Read the model definition and answer for the solid it produces. Units are mm, in the model's axes. A direction names the side the tool comes from. Give positions to 0.01 mm unless a question says otherwise; leave off trailing zeros. Write each loop counter-clockwise with the first axis right and the second up, starting at its lowest first coordinate (ties: lowest second). Pieces come first, ordered by that corner, then holes. Notation, with made-up numbers: (52, -3.75) - (74, -3.75) arc R14 cw to (74, 3.25) - close; hole circle Ø4 at (13, 77). An arc over 180 degrees is marked (long way). Answer as CSV lines item,"result".
```python
from build123d import *

# Parameters (mm, degrees)
F0_W      = 115
F0_H      = 60
F1_DEPTH  = 12
F0_W_2    = 12
F2_DEPTH  = 60
F4_DEPTH  = 25
F5_W      = 50
F5_H      = 20
F6_DEPTH  = 48
F8_DEPTH  = 25
F9_R      = 12.5
F10_DEPTH = 25


with BuildPart() as f1:
    # F0 (on Top) → F1 (new body)
    with BuildSketch(Plane.XY):
        with Locations((-0.438802, -3.920759)):
            Rectangle(F0_W, F0_H)
    extrude(amount=F1_DEPTH)

    # F0 (on Top) → F2 (join)
    with BuildSketch(Plane.XY):
        with Locations((63.061198, -3.920759)):
            Rectangle(F0_W_2, F0_H)
    extrude(amount=F2_DEPTH)

    # F3 (on face) → F4 (cut)
    with BuildSketch(Plane.XY.offset(12)):
        Polygon((57.061198, -33.920759), (-57.938802, 6.079241), (-57.938802, -33.920759), align=None)
    extrude(amount=-F4_DEPTH, mode=Mode.SUBTRACT)

    # F5 (on face) → F6 (join)
    with BuildSketch(Plane.XY.offset(12)):
        with Locations((-32.938802, 16.079241)):
            Rectangle(F5_W, F5_H)
    extrude(amount=F6_DEPTH)

    # F7 (on face) → F8 (cut)
    with BuildSketch(Plane.XZ.offset(-6.079241)):
        with BuildLine():
            Line((-57.938802, 60), (-57.938802, 35))
            ThreePointArc((-57.938802, 35), (-50.616471, 52.67767), (-32.938802, 60))
            Line((-32.938802, 60), (-57.938802, 60))
        make_face()
        with BuildLine():
            Line((-7.938802, 60), (-32.938802, 60))
            ThreePointArc((-32.938802, 60), (-15.261132, 52.67767), (-7.938802, 35))
            Line((-7.938802, 35), (-7.938802, 60))
        make_face()
    extrude(amount=-F8_DEPTH, mode=Mode.SUBTRACT)

    # F9 (on face) → F10 (cut)
    with BuildSketch(Plane.XZ.offset(-6.079241)):
        with Locations((-32.938802, 35)):
            Circle(F9_R)
    extrude(amount=-F10_DEPTH, mode=Mode.SUBTRACT)


solid = f1.part
```
(1) A cutting plane is placed at D-D (z = 51). Write down the section's boundary in (x, y), and give its area (3 significant figures).
Worked out:
outline,"(-52.15, 6.08) - (-13.73, 6.08) - (-13.73, 26.08) - (-52.15, 26.08) - close; (57.06, -33.92) - (69.06, -33.92) - (69.06, 26.08) - (57.06, 26.08) - close"
area,"1,490 mm^2"
(2) A cutting plane is placed at C-C (x = -41.5). Write down the section's boundary in (y, z), and give its area (3 significant figures).
Worked out:
outline,"(0.36, 0) - (26.08, 0) - (26.08, 25.89) - (6.08, 25.89) - (6.08, 12) - (0.36, 12) - close; (6.08, 44.11) - (26.08, 44.11) - (26.08, 58.49) - (6.08, 58.49) - close"
area,"874 mm^2"
(3) Find the intervals of material crossed by L1, parallel to Z at x = 1.5, y = 9.5; L2, parallel to X at y = -6.5, z = 22; L3, parallel to Z at x = -27, y = 16, in increasing order.
Worked out:
L1,"z = 0 to 12"
L2,"x = 57.06 to 69.06"
L3,"z = 0 to 24, 46 to 59.28"
(4) For faces 5 (the flat face through (-44.4, 6.079, 41)), 6 (the flat face through (69.061, -4, 30)), 7 (the flat face through (-7.939, 16, 23)), determine the directions among +Z, -Z, +X, -X, +Y, -Y from which every point of the face is accessible in a straight line to the end or side of a thin tool.
Worked out:
face 5,"+Z, -X, -Y"
face 6,"+Z, -Z, +X, +Y, -Y"
face 7,"+Z, +Y, -Y"
(5) A cutting plane is placed at B-B (z = 31). Write down the section's boundary in (x, y).
Worked out:
outline,"(-57.94, 6.08) - (-44.78, 6.08) - (-44.78, 26.08) - (-57.94, 26.08) - close; (-21.1, 6.08) - (-7.94, 6.08) - (-7.94, 26.08) - (-21.1, 26.08) - close; (57.06, -33.92) - (69.06, -33.92) - (69.06, 26.08) - (57.06, 26.08) - close"
(6) The mould has two halves that part along X. Classify faces 1 (the flat face through (63, -4, 60)), 2 (the flat face through (0.37, -14.2, 6.08)), 3 (the cylindrical face through (-21.392, 15.939, 30.212)), 4 (the flat face through (24, 3, 12)): +X half, -X half, draft (parallel to the pull), parting line (faces both ways), or undercut.
Worked out:
face 1,"draft"
face 2,"-X half"
face 3,"undercut"
face 4,"undercut"
(7) This flat-tipped pin is pushed along its axis until it touches: P1, Ø2, axis at y = 3.5, z = 23, coming from the -X side. Where does it stop, or does it pass through?
Worked out:
P1,"stops at x = 57.06"
(8) A cutting plane is placed at A-A (y = 15). Write down the section's boundary in (x, z).
Worked out:
outline,"(-57.94, 0) - (69.06, 0) - (69.06, 60) - (57.06, 60) - (57.06, 12) - (-7.94, 12) - (-7.94, 35) arc R25 ccw to (-32.94, 60) arc R25 ccw to (-57.94, 35) - close; hole circle Ø25 at (-32.94, 35)"
